CAD build for the part. Positions are in the model's coordinates, mm. A direction names the side the tool comes from. Coordinates: 2 decimals unless noted, no trailing zeros. Order: outer loops, then holes, each group sorted by start corner. A loop starts at its lowest first (then second) coordinate and runs counter-clockwise, first axis right, second up. Notation, with made-up numbers: (-21, 73) - (-1, 73) arc R22 cw to (-1, 100) - close; hole circle Ø9 at (22, 52). An arc over 180 degrees is marked (long way). Use one line per item in the form item = value.
```python
from build123d import *

# Parameters (mm, degrees)
F0_R     = 0.4
F1_DEPTH = 1.4
F2_DEPTH = 2.3
F3_DEPTH = 0.5


with BuildPart() as f1:
    # F0 (on Top) → F1 (new body)
    with BuildSketch(Plane.XY):
        with BuildLine():
            ThreePointArc((2.7, -2.1476731595), (3.2571076126, -1.1374313166), (3.45, 0))
            ThreePointArc((3.45, 0), (3.2571076126, 1.1374313166), (2.7, 2.1476731595))
            Line((2.7, 2.1476731595), (1.0139649895, 2.1476731595))
            ThreePointArc((1.0139649895, 2.1476731595), (2.0060897101, 1.2713099838), (2.375, 0))
            ThreePointArc((2.375, 0), (2.0060897101, -1.2713099838), (1.0139649895, -2.1476731595))
            Line((1.0139649895, -2.1476731595), (2.7, -2.1476731595))
        make_face()
        with BuildLine():
            Line((1.0139649895, 2.1476731595), (2.7, 2.1476731595))
            ThreePointArc((2.7, 2.1476731595), (0, 3.45), (-2.7, 2.1476731595))
            Line((-2.7, 2.1476731595), (-1.0139649895, 2.1476731595))
            ThreePointArc((-1.0139649895, 2.1476731595), (0, 2.375), (1.0139649895, 2.1476731595))
        make_face()
        with BuildLine():
            ThreePointArc((-2.7, 2.1476731595), (0, 3.45), (2.7, 2.1476731595))
            Line((2.7, 2.1476731595), (2.0471920173, 14.6072606371))
            ThreePointArc((2.0471920173, 14.6072606371), (2.0492978841, 14.553648693), (2.05, 14.5))
            ThreePointArc((2.05, 14.5), (-0.053648693, 12.4507021159), (-2.0471920173, 14.6072606371))
            Line((-2.0471920173, 14.6072606371), (-2.7, 2.1476731595))
        make_face()
        with BuildLine():
            Line((2.0471920173, -14.6072606371), (2.7, -2.1476731595))
            ThreePointArc((2.7, -2.1476731595), (0, -3.45), (-2.7, -2.1476731595))
            Line((-2.7, -2.1476731595), (-2.0471920173, -14.6072606371))
            ThreePointArc((-2.0471920173, -14.6072606371), (-0.053648693, -12.4507021159), (2.05, -14.5))
            ThreePointArc((2.05, -14.5), (2.0492978841, -14.553648693), (2.0471920173, -14.6072606371))
        make_face()
        with BuildLine():
            ThreePointArc((-2.7, -2.1476731595), (0, -3.45), (2.7, -2.1476731595))
            Line((2.7, -2.1476731595), (1.0139649895, -2.1476731595))
            ThreePointArc((1.0139649895, -2.1476731595), (0, -2.375), (-1.0139649895, -2.1476731595))
            Line((-1.0139649895, -2.1476731595), (-2.7, -2.1476731595))
        make_face()
        with BuildLine():
            Line((-1.0139649895, 2.1476731595), (-2.7, 2.1476731595))
            ThreePointArc((-2.7, 2.1476731595), (-3.45, 0), (-2.7, -2.1476731595))
            Line((-2.7, -2.1476731595), (-1.0139649895, -2.1476731595))
            ThreePointArc((-1.0139649895, -2.1476731595), (-2.375, 0), (-1.0139649895, 2.1476731595))
        make_face()
        with BuildLine():
            ThreePointArc((2.05, 14.5), (2.0492978841, 14.553648693), (2.0471920173, 14.6072606371))
            ThreePointArc((2.0471920173, 14.6072606371), (0, 16.55), (-2.0471920173, 14.6072606371))
            ThreePointArc((-2.0471920173, 14.6072606371), (-0.053648693, 12.4507021159), (2.05, 14.5))
        make_face()
        with Locations((0, 14.5)):
            Circle(F0_R, mode=Mode.SUBTRACT)
        with BuildLine():
            ThreePointArc((-2.0471920173, -14.6072606371), (0, -16.55), (2.0471920173, -14.6072606371))
            ThreePointArc((2.0471920173, -14.6072606371), (2.0492978841, -14.553648693), (2.05, -14.5))
            ThreePointArc((2.05, -14.5), (-0.053648693, -12.4507021159), (-2.0471920173, -14.6072606371))
        make_face()
        with Locations((0, -14.5)):
            Circle(F0_R, mode=Mode.SUBTRACT)
    extrude(amount=F1_DEPTH)

    # F0 (on Top) → F2 (join)
    with BuildSketch(Plane.XY):
        with BuildLine():
            Line((-1.0139649895, 2.1476731595), (-2.7, 2.1476731595))
            ThreePointArc((-2.7, 2.1476731595), (-3.45, 0), (-2.7, -2.1476731595))
            Line((-2.7, -2.1476731595), (-1.0139649895, -2.1476731595))
            ThreePointArc((-1.0139649895, -2.1476731595), (-2.375, 0), (-1.0139649895, 2.1476731595))
        make_face()
        with BuildLine():
            Line((1.0139649895, 2.1476731595), (2.7, 2.1476731595))
            ThreePointArc((2.7, 2.1476731595), (0, 3.45), (-2.7, 2.1476731595))
            Line((-2.7, 2.1476731595), (-1.0139649895, 2.1476731595))
            ThreePointArc((-1.0139649895, 2.1476731595), (0, 2.375), (1.0139649895, 2.1476731595))
        make_face()
        with BuildLine():
            ThreePointArc((-2.7, -2.1476731595), (0, -3.45), (2.7, -2.1476731595))
            Line((2.7, -2.1476731595), (1.0139649895, -2.1476731595))
            ThreePointArc((1.0139649895, -2.1476731595), (0, -2.375), (-1.0139649895, -2.1476731595))
            Line((-1.0139649895, -2.1476731595), (-2.7, -2.1476731595))
        make_face()
        with BuildLine():
            ThreePointArc((2.7, -2.1476731595), (3.2571076126, -1.1374313166), (3.45, 0))
            ThreePointArc((3.45, 0), (3.2571076126, 1.1374313166), (2.7, 2.1476731595))
            Line((2.7, 2.1476731595), (1.0139649895, 2.1476731595))
            ThreePointArc((1.0139649895, 2.1476731595), (2.0060897101, 1.2713099838), (2.375, 0))
            ThreePointArc((2.375, 0), (2.0060897101, -1.2713099838), (1.0139649895, -2.1476731595))
            Line((1.0139649895, -2.1476731595), (2.7, -2.1476731595))
        make_face()
    extrude(amount=-F2_DEPTH)

    # F0 (on Top) → F3 (join)
    with BuildSketch(Plane.XY):
        with BuildLine():
            Line((0, 2.1476731595), (1.0139649895, 2.1476731595))
            ThreePointArc((1.0139649895, 2.1476731595), (0, 2.375), (-1.0139649895, 2.1476731595))
            Line((-1.0139649895, 2.1476731595), (0, 2.1476731595))
        make_face()
        with BuildLine():
            ThreePointArc((2.375, 0), (2.0060897101, 1.2713099838), (1.0139649895, 2.1476731595))
            Line((1.0139649895, 2.1476731595), (0, 2.1476731595))
            Line((0, 2.1476731595), (-1.0139649895, 2.1476731595))
            ThreePointArc((-1.0139649895, 2.1476731595), (-2.375, 0), (-1.0139649895, -2.1476731595))
            Line((-1.0139649895, -2.1476731595), (1.0139649895, -2.1476731595))
            ThreePointArc((1.0139649895, -2.1476731595), (2.0060897101, -1.2713099838), (2.375, 0))
        make_face()
        with BuildLine():
            ThreePointArc((1.175, 0), (-0.8308504679, -0.8308504679), (0, 1.175))
            ThreePointArc((0, 1.175), (0.8308504679, 0.8308504679), (1.175, 0))
        make_face(mode=Mode.SUBTRACT)
        with BuildLine():
            ThreePointArc((-1.0139649895, -2.1476731595), (0, -2.375), (1.0139649895, -2.1476731595))
            Line((1.0139649895, -2.1476731595), (-1.0139649895, -2.1476731595))
        make_face()
    extrude(amount=F3_DEPTH)


solid = f1.part
```
Item 1: Drill centre lines: line 1 (Z direction, x = 1.75, y = -8); line 2 (Y direction, x = 1.5, z = -0.3); line 3 (Z direction, x = 0, y = 1.5). Where is each one in solid material? Low to high. Write a range as [from, to].
Derived:
line_1 = [0, 1.4]
line_2 = [-3.11, -1.84], [1.84, 3.11]
line_3 = [0, 0.5]
Item 2: Cut at A-A, the plane z = 1.05. Write the cut outline in (x, y) (3 decimals), plus the area to 3 significant figures.
Derived:
outline = (-2.7, -2.148) - (-2.047, -14.607) arc R2.05 ccw to (2.047, -14.607) - (2.7, -2.148) arc R3.45 ccw to (2.7, 2.148) - (2.047, 14.607) arc R2.05 ccw to (-2.047, 14.607) - (-2.7, 2.148) arc R3.45 ccw to start; hole circle Ø4.75 at (0, 0); hole circle Ø0.8 at (0, -14.5); hole circle Ø0.8 at (0, 14.5)
area = 139 mm²
Item 3: Cut at B-B, the plane z = -0.6. Write the cut outline in (x, y) (3 decimals).
Derived:
outline = circle Ø6.9 at (0, 0); hole circle Ø4.75 at (0, 0)
Item 4: Cut at C-C, the plane x = -1.5. Write the cut outline in (y, z), plus the area to 3 significant figures.
Derived:
outline = (-15.9, 0) - (-3.11, 0) - (-3.11, -2.3) - (-1.84, -2.3) - (-1.84, 0) - (1.84, 0) - (1.84, -2.3) - (3.11, -2.3) - (3.11, 0) - (15.9, 0) - (15.9, 1.4) - (1.84, 1.4) - (1.84, 0.5) - (-1.84, 0.5) - (-1.84, 1.4) - (-15.9, 1.4) - close
area = 47.0 mm²
Item 5: 3-axis set-ups, long thin cutter, end or side, ignore diameter. For faces 1 (the face through (-1, 1, 0)), 2 (the face through (-2.37, 8.46, 0.69)), 3 (the face through (-1, 1, 0.5)): which of +Z, -Z, +X, -X, +Y, -Y reach the whole face in a straight line?
Derived:
face_1 = -Z
face_2 = +Z, -Z, -X, +Y
face_3 = +Z
Item 6: Cut at D-D, the plane y = 12.5. Write the cut outline in (x, z), plus the area to 3 significant figures.
Derived:
outline = (-2.16, 0) - (2.16, 0) - (2.16, 1.4) - (-2.16, 1.4) - close
area = 6.04 mm²
Item 7: Drop flat-ended pins along their axis: pin 1 (3 mm diameter, centred on x = -1.5, y = 5.5, fed in from -Z); pin 2 (1.4 mm diameter, centred on x = 0, y = 0, fed in from +Z). Give the stop position or say it passes through.
Derived:
pin_1 = 0
pin_2 = through
Item 8: Two-plate mould, pull along X, no slides. Class faces 4 (the face through (2.37, -8.46, 0.69)), 5 (the face through (-0.04, -16.55, 0.69)), 6 (the face through (0, -9, 0)), 7 (the face through (0.215, -14.163, 0.69)): +X half, -X half, draft (parallel to the pull), parting line (faces both ways), or undercut.
Derived:
face_4 = +X half
face_5 = parting line
face_6 = draft
face_7 = undercut
